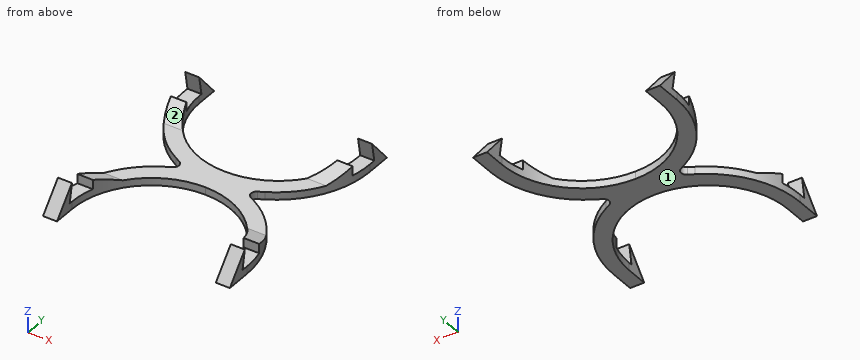
```python
from build123d import *

# Parameters (mm, degrees)
F1_DEPTH = 50
F4_DEPTH = 14.001
F6_DEPTH = 4
F7_R     = 50
F8_R     = 3


# Not quite as in the source:
# - a pattern or mirror of a feature is missing from the dataset's text; its kind, count and spacing are read off the source's solid


with BuildPart() as f1:
    # F0 (on Right) → F1 (new body, symmetric)
    with BuildSketch(Plane.YZ):
        Polygon((0, 4), (0, 0), (61.7473948365, 0), (50, 14), (51.7632698071, 4), (36.7632698071, 4), (36.7632698071, 9), (23.5265396142, 4), align=None)
    extrude(amount=F1_DEPTH, both=True)

    # F2: F1 across face


with BuildPart() as f1_1:
    add(f1.part)
    add(f1.part.mirror(Plane(origin=(0, 0, 2), x_dir=(1, 0, 0), z_dir=(0, -1, 0))))

    # F3 (on face) → F4 (cut, through all)
    with BuildSketch(Plane(origin=(0, 0, 0), x_dir=(1, 0, 0), z_dir=(0, 0, -1))):
        with BuildLine():
            Line((42.5, 50), (42.5, 61.7473948365))
            Line((42.5, 61.7473948365), (0, 61.7473948365))
            Line((0, 61.7473948365), (-42.5, 61.7473948365))
            Line((-42.5, 61.7473948365), (-42.5, 50))
            ThreePointArc((-42.5, 50), (-30.0520382004, 19.9479617996), (0, 7.5))
            ThreePointArc((0, 7.5), (30.0520382004, 19.9479617996), (42.5, 50))
        make_face()
    f4 = extrude(amount=-F4_DEPTH, mode=Mode.SUBTRACT)

    # F4_copies: F4 across plane
    add(f4.mirror(Plane.ZX), mode=Mode.SUBTRACT)

    # F5 (on face) → F6 (cut, through all)
    with BuildSketch(Plane.XY.offset(4)):
        Polygon((-50, 18.5265396142), (-50, -18.5265396142), (-16.0078105936, 0), align=None)
        Polygon((50, 18.5265396142), (16.0078105936, 0), (50, -18.5265396142), align=None)
    extrude(amount=-F6_DEPTH, mode=Mode.SUBTRACT)

    # F7
    f7_edges = [f1_1.edges().sort_by_distance(p)[0] for p in [
        (50, -18.52654, 2),
        (50, 18.52654, 2),
        (-50, -18.52654, 2),
        (-50, 18.52654, 2),
    ]]
    fillet(f7_edges, radius=F7_R)

    # F8
    f8_edges = [f1_1.edges().sort_by_distance(p)[0] for p in [
        (-16.007811, 0, 2),
        (16.007811, 0, 2),
    ]]
    fillet(f8_edges, radius=F8_R)


solid = f1_1.part
```
Source: CAD feature listing. Evaluate the final solid. Frame: model axes, mm. Face numbers are marked on the shaded views. A direction names the side the tool comes from. Round coordinates to 2 decimals unless told otherwise and drop trailing zeros. Loops run counter-clockwise (first coordinate to the right, second up) from the corner with the lowest first, then second, coordinate; pieces in that order, holes last.
1. Section query D-D on z = 1.5. Output: boundary loops of the cut face in (x, y).
2. Section query A-A on z = 10.75. Output: boundary loops of the cut face in (x, y).
3. Contact query for flat-ended pins moving along their axis: pin 1 (5 mm diameter, centred on x = -44, y = 41.5, fed in from +Z); pin 2 (5.5 mm diameter, centred on x = -43.5, z = 7.5, fed in from +Y); pin 3 (2 mm diameter, centred on y = -44.5, z = 3, fed in from -X). Output: stop coordinate, or through.
4. Ray query, L1, parallel to X at y = 53, z = 5; L2, parallel to Z at x = 17, y = 4; L3, parallel to X at y = -29.5, z = 5. Return the intervals inside material, ascending.
5. Section query C-C on y = 18.5. Output: boundary loops of the cut face in (x, z), and give its area (3 significant figures).
6. Access query for the marked faces 1 and 2. Directions: +Z, -Z, +X, -X, +Y, -Y. A direction counts if a zero-diameter tool reaches every point of the face in a straight line with its end or side. Return the directions, or none.
7. Section query B-B on y = -41. Output: boundary loops of the cut face in (x, z).
Answers below:
1. outline: (-50, -60.49) - (-42.5, -60.49) - (-42.5, -50) arc R42.5 cw to (42.5, -50) - (42.5, -60.49) - (50, -60.49) - (50, -48.22) arc R50 ccw to (23.93, -4.32) - (20.84, -2.63) arc R3 cw to (20.84, 2.63) - (23.93, 4.32) arc R50 ccw to (50, 48.22) - (50, 60.49) - (42.5, 60.49) - (42.5, 50) arc R42.5 cw to (-42.5, 50) - (-42.5, 60.49) - (-50, 60.49) - (-50, 48.22) arc R50 ccw to (-23.93, 4.32) - (-20.84, 2.63) arc R3 cw to (-20.84, -2.63) - (-23.93, -4.32) arc R50 ccw to (-50, -48.22) - close
2. outline: (-50, -52.73) - (-42.5, -52.73) - (-42.5, -50.57) - (-50, -50.57) - close; (-50, 50.57) - (-42.5, 50.57) - (-42.5, 52.73) - (-50, 52.73) - close; (42.5, -52.73) - (50, -52.73) - (50, -50.57) - (42.5, -50.57) - close; (42.5, 50.57) - (50, 50.57) - (50, 52.73) - (42.5, 52.73) - close
3. pin 1: stops at z = 4
3. pin 2: stops at y = 57.76
3. pin 3: stops at x = -49.93
4. L1: x = -50 to -42.5, 42.5 to 50
4. L2: z = 0 to 4
4. L3: x = -46.36 to -37.23, 37.23 to 46.36
5. outline: (-40.21, 0) - (-28.53, 0) - (-28.53, 4) - (-40.21, 4) - close; (28.53, 0) - (40.21, 0) - (40.21, 4) - (28.53, 4) - close
5. area: 93.4 mm2
6. face 1: -Z, +X, -X, +Y, -Y
6. face 2: +Z, +X, -X
7. outline: (-49.48, 0) - (-41.54, 0) - (-41.54, 4) - (-49.48, 4) - close; (41.54, 0) - (49.48, 0) - (49.48, 4) - (41.54, 4) - close
